Could you check a few things on this model? Use its own coordinates, in mm. Face numbers are marked on the shaded views. A direction names the side the tool comes from. Give positions to 0.01 mm unless a question says otherwise; leave off trailing zeros. Order: outer loops, then holes, each group sorted by start corner. A loop starts at its lowest first (then second) coordinate and runs counter-clockwise, first axis right, second up. Notation, with made-up numbers: M 13,-6.5 L 31,-6.5 A19 ccw 31,25.5 Z; hole C 0,-22.75 d7. An arc over 180 degrees is marked long. Use a Markdown table: item, result. Add a question column.
```python
from build123d import *

# Parameters (mm, degrees)
SKETCH1_W           = 22.75
SKETCH1_H           = 11.5
BOSS_EXTRUDE1_DEPTH = 16
BOSS_EXTRUDE2_DEPTH = 11.5
SKETCH3_R           = 5.5
BOSS_EXTRUDE3_DEPTH = 4.5
FILLET1_R           = 1
SKETCH5_R           = 2.25
BOSS_EXTRUDE5_DEPTH = 3
SKETCH6_R           = 0.75
CUT_EXTRUDE1_DEPTH  = 5
CUT_EXTRUDE2_START  = -0.5
CUT_EXTRUDE2_DEPTH  = 10
SKETCH7_R           = 2
CUT_EXTRUDE3_DEPTH  = 36.01874498


with BuildPart() as part:
    # Sketch1 → Boss-Extrude1 (new body)
    with BuildSketch(Plane(origin=(0, 0, 0), x_dir=(1, 0, 0), z_dir=(0, 1, 0))):
        with Locations((11.375, 5.75)):
            Rectangle(SKETCH1_W, SKETCH1_H)
    extrude(amount=BOSS_EXTRUDE1_DEPTH)

    # Sketch2 → Boss-Extrude2 (add)
    with BuildSketch(Plane.XY):
        Polygon((22.75, 16), (27.75, 16), (27.75, 18), (25.25, 18), (22.75, 20.5), (16.75, 22), (0, 22), (0, 20.5), (-2.5, 18), (-5, 18), (-5, 16), (0, 16), align=None)
    extrude(amount=-BOSS_EXTRUDE2_DEPTH)

    # Sketch3 → Boss-Extrude3 (add)
    with BuildSketch(Plane(origin=(0, 22, 0), x_dir=(1, 0, 0), z_dir=(0, 1, 0))):
        with Locations(Location((5.5, 5.75, 0), (0, 0, 180))):
            Circle(SKETCH3_R)
    extrude(amount=BOSS_EXTRUDE3_DEPTH)

    # Fillet1
    fillet1_edges = [part.edges().sort_by_distance(p)[0] for p in [
        (11, 26.5, -5.75),
    ]]
    fillet(fillet1_edges, radius=FILLET1_R)

    # Sketch5 → Boss-Extrude5 (add)
    with BuildSketch(Plane(origin=(0, 26.5, 0), x_dir=(1, 0, 0), z_dir=(0, 1, 0))):
        with Locations(Location((5.5, 5.75, 0), (0, 0, 180))):
            Circle(SKETCH5_R)
    extrude(amount=BOSS_EXTRUDE5_DEPTH)

    # Sketch6 → Cut-Extrude1 (cut)
    with BuildSketch(Plane(origin=(0, 29.5, 0), x_dir=(1, 0, 0), z_dir=(0, 1, 0))):
        with Locations(Location((5.5, 5.75, 0), (0, 0, 180))):
            Circle(SKETCH6_R)
    extrude(amount=-CUT_EXTRUDE1_DEPTH, mode=Mode.SUBTRACT)

    # Sketch8 → Cut-Extrude2 (cut)
    with BuildSketch(Plane.XY.offset(CUT_EXTRUDE2_START)):
        Polygon((-2.5, 18), (0, 18), (0, 20.5), align=None)
        Polygon((22.75, 20.5), (22.75, 18), (25.25, 18), align=None)
    extrude(amount=-CUT_EXTRUDE2_DEPTH, mode=Mode.SUBTRACT)

    # Sketch7 → Cut-Extrude3 (cut, through all)
    with BuildSketch(Plane(origin=(0, 18, 0), x_dir=(1, 0, 0), z_dir=(0, 1, 0))):
        with Locations((26.25, 5.5)):
            Circle(SKETCH7_R)
        with Locations((-3.5, 5.5)):
            Circle(SKETCH7_R)
    extrude(amount=-CUT_EXTRUDE3_DEPTH, mode=Mode.SUBTRACT)


solid = part.part
```
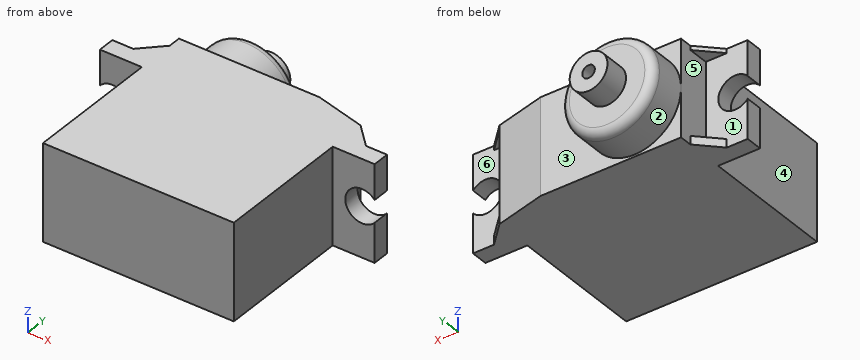
1) We'd pull the mould along Z, two halves only. Please class the marked faces 1, 2 and 3: pulls with the +Z half, pulls with the -Z half, needs draft (parallel to the pull), parting line crosses it, or undercut.
2) For the marked faces 4, 5 and 6, which set-ups out of +Z, -Z, +X, -X, +Y, -Y let a thin tool reach every point of the face, with its end or its side?
3) Suppose I cut it at A-A on x = -3.5. Please give me the cut outline in (y, z), and give its area (3 significant figures).
4) For pin 1 (1.5 mm diameter, centred on y = 5.5, z = -4, fed in from +X); pin 2 (6 mm diameter, centred on x = 21.5, z = -2.5, fed in from +Y); pin 3 (4.5 mm diameter, centred on x = 4, z = -7.5, fed in from +Y); pin 4 (1.4 mm diameter, centred on x = 5.5, z = -5.75, fed in from +Y), each with a flat end and sliding along its axis, tell me the tip position at first contact or that it passes through.
5) Please list where these lines run through material, in increasing order: line 1 (Z direction, x = 26.25, y = 16.7); line 2 (Y direction, x = 4, z = -3.75); line 3 (Y direction, x = 23.5, z = -2.75). Write a range as from..to.
6) Suppose I cut it at C-C on y = 27.5. Please give me the cut outline in (x, z), and give its area (3 significant figures).
7) Suppose I cut it at D-D on y = 5.5. Please give me the cut outline in (x, z).
8) Suppose I cut it at B-B on x = 5.5. Please give me the cut outline in (y, z), and give its area (3 significant figures).
Values found:
| question | item | result |
|---|---|---|
| 1 | face 1 | undercut |
| 1 | face 2 | parting line crosses it |
| 1 | face 3 | needs draft |
| 2 | face 4 | +Z, -Z, -X, -Y |
| 2 | face 5 | -X, +Y |
| 2 | face 6 | +X, +Y |
| 3 | outline | M 16,-11.5 L 18,-11.5 L 18,-7.5 L 16,-7.5 Z; M 16,-3.5 L 18,-3.5 L 18,0 L 16,0 Z |
| 3 | area | 15.0 mm^2 |
| 4 | pin 1 | stops at x = 22.75 |
| 4 | pin 2 | stops at y = 21.56 |
| 4 | pin 3 | stops at y = 29.5 |
| 4 | pin 4 | stops at y = 24.5 |
| 5 | line 1 | z = -11.5..-7.5, -3.5..0 |
| 5 | line 2 | y = 0..26.5 |
| 5 | line 3 | y = 16..18 |
| 6 | outline | C 5.5,-5.75 d4.5; hole C 5.5,-5.75 d1.5 |
| 6 | area | 14.1 mm^2 |
| 7 | outline | M 0,-11.5 L 22.75,-11.5 L 22.75,0 L 0,0 Z |
| 8 | outline | M 0,-11.5 L 22,-11.5 L 22,-11.25 L 25.5,-11.25 A1 ccw 26.5,-10.25 L 26.5,-8 L 29.5,-8 L 29.5,-6.5 L 24.5,-6.5 L 24.5,-5 L 29.5,-5 L 29.5,-3.5 L 26.5,-3.5 L 26.5,-1.25 A1 ccw 25.5,-0.25 L 22,-0.25 L 22,0 L 0,0 Z |
| 8 | area | 308 mm^2 |
